Design review of the part built by this model. Coordinates are the model's own, in mm. A direction names the side the tool comes from. Coordinates: 2 decimals unless noted, no trailing zeros. Order: outer loops, then holes, each group sorted by start corner. A loop starts at its lowest first (then second) coordinate and runs counter-clockwise, first axis right, second up.
from build123d import *

# Parameters (mm, degrees)
BOSS_EXTRUDE1_DEPTH = 4
SKETCH2_R           = 2.1
CUT_EXTRUDE1_DEPTH  = 19.812296511
SKETCH3_W           = 40
SKETCH3_H           = 10
CUT_EXTRUDE2_DEPTH  = 0.6
CHAMFER1_SIZE       = 2


with BuildPart() as part:
    # Sketch1 → Boss-Extrude1 (new, symmetric)
    with BuildSketch(Plane.XY):
        with BuildLine():
            Line((-4.05, 0), (-16, 0))
            Line((-16, 0), (-16, 3))
            Line((-16, 3), (-8.538296083, 3))
            ThreePointArc((-8.538296083, 3), (0, 9.05), (8.538296083, 3))
            Line((8.538296083, 3), (16, 3))
            Line((16, 3), (16, 0))
            Line((16, 0), (4.05, 0))
            ThreePointArc((4.05, 0), (0, 4.05), (-4.05, 0))
        make_face()
    extrude(amount=BOSS_EXTRUDE1_DEPTH, both=True)

    # Sketch2 → Cut-Extrude1 (cut, through all)
    with BuildSketch(Plane(origin=(0, 0, 0), x_dir=(1, 0, 0), z_dir=(0, 1, 0))):
        with Locations((-12, 0)):
            Circle(SKETCH2_R)
        with Locations((12, 0)):
            Circle(SKETCH2_R)
    extrude(amount=CUT_EXTRUDE1_DEPTH, mode=Mode.SUBTRACT)

    # Sketch3 → Cut-Extrude2 (cut)
    with BuildSketch(Plane(origin=(0, 0, 0), x_dir=(1, 0, 0), z_dir=(0, 1, 0))):
        Rectangle(SKETCH3_W, SKETCH3_H)
    extrude(amount=CUT_EXTRUDE2_DEPTH, mode=Mode.SUBTRACT)

    # Chamfer1
    chamfer1_edges = [part.edges().sort_by_distance(p)[0] for p in [
        (-16, 1.8, 4),
        (16, 1.8, -4),
        (16, 1.8, 4),
        (-16, 1.8, -4),
    ]]
    chamfer(chamfer1_edges, length=CHAMFER1_SIZE)


solid = part.part
1. Add section C-C (y = 1.5). Give the boundary of the cut face in (x, z).
2. Add section A-A (x = 12). Give the boundary of the cut face in (y, z), and give its area (3 significant figures).
3. To check wall thickness, follow line 1 (Z direction, x = -12, y = 1.7); line 2 (X direction, y = 2.5, z = -0.75); line 3 (Y direction, x = -9.5, z = -2.25). State the ranges of each line that lie inside material, in increasing order.
4. Mouldability with a two-part tool opening along Z and no side actions: class faces 4 (the cylindrical face through (-14.1, 1.78, -0.09)), 5 (the flat face through (15, 2, 3)), 6 (the flat face through (-15, 2, -3)) as pulls with the +Z half, pulls with the -Z half, needs draft (parallel to the pull), parting line crosses it, or undercut.
5. Add section D-D (x = -13.5). Give the boundary of the cut face in (y, z), and give its area (3 significant figures).
6. For faces 1 (the flat face through (9.7, 3, 0.1)), 2 (the flat face through (9, 0.6, 0)), 3 (the flat face through (-10.66, 3, 1.83)), list the 3-axis set-ups (+Z, -Z, +X, -X, +Y, -Y) from which the entire face can be reached by the end or side of a thin tool; tool diameter is ignored.
7. Add section B-B (z = 0). Give the boundary of the cut face in (x, y).
8. Insertion check: pin 1 (1 mm diameter, centred on x = 12, z = -2, fed in from -Y); pin 2 (2.5 mm diameter, centred on x = 12, z = 0, fed in from -Y); pin 3 (1 mm diameter, centred on y = 5.5, z = 0.5, fed in from +X); pin 4 (2 mm diameter, centred on y = 7.5, z = 1, fed in from -X). Each pin has a flat end and moves straight along its axis. Give the tip position at first contact, or say it passes through.
Solution:
1. outline: (-16, -2) - (-14, -4) - (-3.76, -4) - (-3.76, 4) - (-14, 4) - (-16, 2) - close; (3.76, -4) - (14, -4) - (16, -2) - (16, 2) - (14, 4) - (3.76, 4) - close; hole circle Ø4.2 at (-12, 0); hole circle Ø4.2 at (12, 0)
2. outline: (0.6, -4) - (3, -4) - (3, -2.1) - (0.6, -2.1) - close; (0.6, 2.1) - (3, 2.1) - (3, 4) - (0.6, 4) - close
2. area: 9.12 mm2
3. line 1: z = -4 to -2.1, 2.1 to 4
3. line 2: x = -16 to -13.96, -10.04 to -3.19, 3.19 to 10.04, 13.96 to 16
3. line 3: y = 0.6 to 3
4. face 4: undercut
4. face 5: pulls with the +Z half
4. face 6: pulls with the -Z half
5. outline: (0.6, -4) - (3, -4) - (3, -1.47) - (0.6, -1.47) - close; (0.6, 1.47) - (3, 1.47) - (3, 4) - (0.6, 4) - close
5. area: 12.1 mm2
6. face 1: +Z, -Z, +X, +Y
6. face 2: +Z, -Z, +X, -X, -Y
6. face 3: +Z, -Z, -X, +Y
7. outline: (-16, 0.6) - (-14.1, 0.6) - (-14.1, 3) - (-16, 3) - close; (-9.9, 0.6) - (-4.01, 0.6) arc R4.05 cw to (4.01, 0.6) - (9.9, 0.6) - (9.9, 3) - (8.54, 3) arc R9.05 ccw to (-8.54, 3) - (-9.9, 3) - close; (14.1, 0.6) - (16, 0.6) - (16, 3) - (14.1, 3) - close
8. pin 1: stops at y = 0.6
8. pin 2: passes through
8. pin 3: stops at x = 7.54
8. pin 4: stops at x = -6.3
